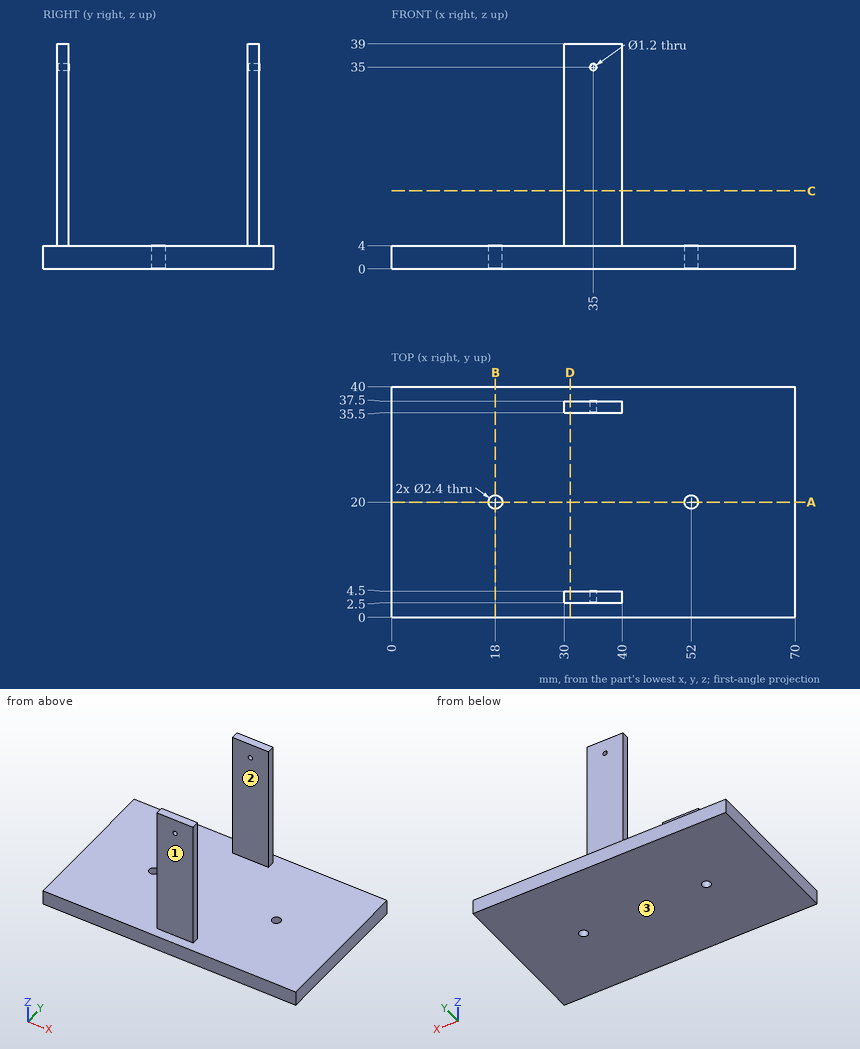
Part print with two shaded views. Sizes in mm from the minimum x, y, z corner. Give positions to 0.01 mm unless a question says otherwise; leave off trailing zeros. Order: outer loops, then holes, each group sorted by start corner. A loop starts at its lowest first (then second) coordinate and runs counter-clockwise, first axis right, second up.
1) Saw through at A-A, the plane y = 20. Write the cut outline in (x, z), then the cut area to 3 significant figures.
2) Pin check, flat tips, straight feed: pin 1 (1.4 mm diameter, centred on x = 35, z = 35, fed in from -Y); pin 2 (1.4 mm diameter, centred on x = 35, z = 35, fed in from +Y); pin 3 (0.6 mm diameter, centred on y = 36.5, z = 29.5, fed in from +X). Stop position of each tip, or through.
3) Saw through at B-B, the plane x = 18. Write the cut outline in (y, z), then the cut area to 3 significant figures.
4) Wall check: probe 1 along X at (y, z) = (20, 0.8); probe 2 along Z at (x, y) = (35, 3.35); probe 3 along X at (y, z) = (36.7, 35). Give the ranges that are in metal, low to high.
5) Saw through at D-D, the plane x = 31. Write the cut outline in (y, z), then the cut area to 3 significant figures.
6) Mould opens along Y. For the marked faces 1, 2 and 3 say: +Y half, -Y half, draft (parallel to the pull), parting line (faces both ways), or undercut.
7) Saw through at C-C, the plane z = 13.5. Write the cut outline in (x, y).
Computed:
1. outline: (0, 0) - (16.8, 0) - (16.8, 4) - (0, 4) - close; (19.2, 0) - (50.8, 0) - (50.8, 4) - (19.2, 4) - close; (53.2, 0) - (70, 0) - (70, 4) - (53.2, 4) - close
1. area: 261 mm2
2. pin 1: stops at y = 2.5
2. pin 2: stops at y = 37.5
2. pin 3: stops at x = 40
3. outline: (0, 0) - (18.8, 0) - (18.8, 4) - (0, 4) - close; (21.2, 0) - (40, 0) - (40, 4) - (21.2, 4) - close
3. area: 150 mm2
4. probe 1: x = 0 to 16.8, 19.2 to 50.8, 53.2 to 70
4. probe 2: z = 0 to 34.4, 35.6 to 39
4. probe 3: x = 30 to 34.4, 35.6 to 40
5. outline: (0, 0) - (40, 0) - (40, 4) - (37.5, 4) - (37.5, 39) - (35.5, 39) - (35.5, 4) - (4.5, 4) - (4.5, 39) - (2.5, 39) - (2.5, 4) - (0, 4) - close
5. area: 300 mm2
6. face 1: -Y half
6. face 2: undercut
6. face 3: draft
7. outline: (30, 2.5) - (40, 2.5) - (40, 4.5) - (30, 4.5) - close; (30, 35.5) - (40, 35.5) - (40, 37.5) - (30, 37.5) - close
